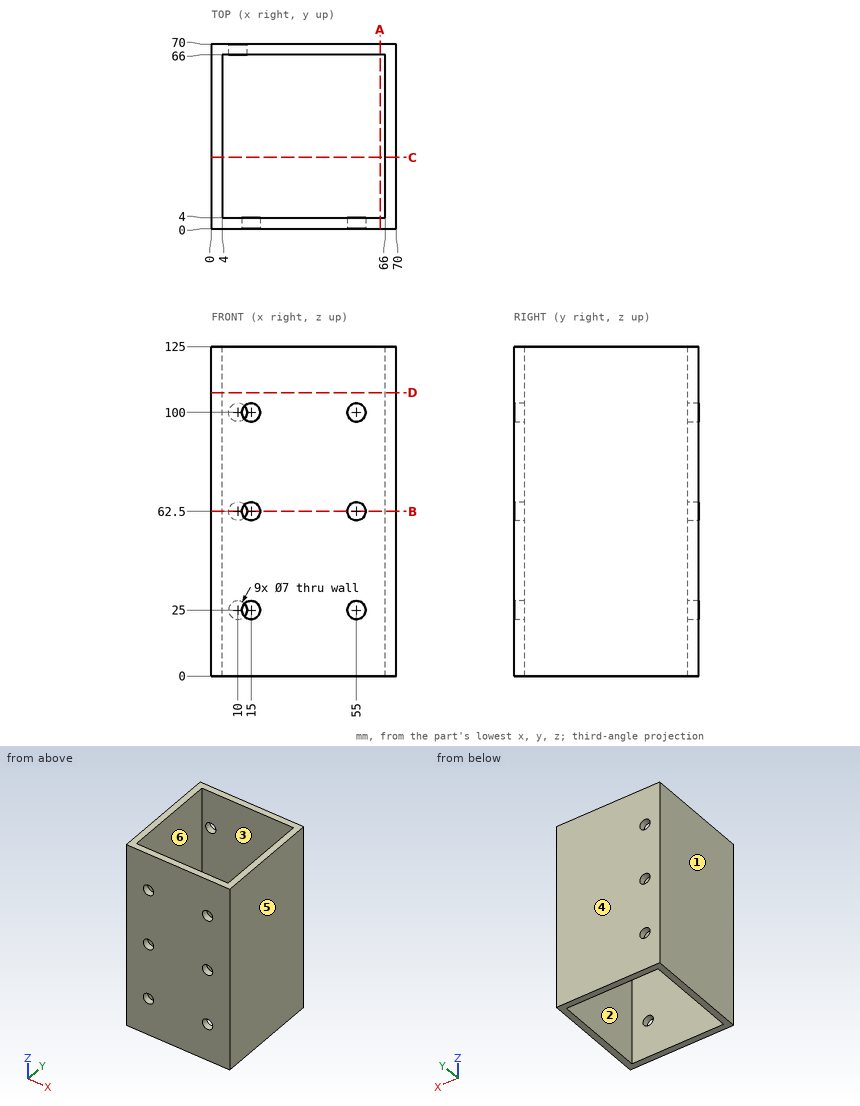
Part print with two shaded views. Sizes in mm from the minimum x, y, z corner. A direction names the side the tool comes from. Coordinates: 2 decimals unless noted, no trailing zeros. Loops run counter-clockwise (first coordinate to the right, second up) from the corner with the lowest first, then second, coordinate; pieces in that order, holes last. Notation, with made-up numbers: (59, 83) -> (101, 83) arc R27 ccw to (101, 104) -> close; hole circle Ø7 at (8, 11). An arc over 180 degrees is marked (long way). Answer as a JSON object with one key per item and string values.
Q1. Flat gauge pins, fed straight in: P1, Ø4, axis at x = 55, z = 62.5, coming from the -Y side; P2, Ø3, axis at x = 42, z = 91.5, coming from the -Y side; P3, Ø10, axis at x = 56.5, y = 50, coming from the +Z side. Where does each tip first touch, or does it go through?
Report:
{"P1": "stops at y = 66", "P2": "stops at y = 0", "P3": "passes through"}
Q2. Probe probe 1 along Z at (x, y) = (15, 2.45); probe 2 along Y at (x, z) = (12, 35); probe 3 along X at (y, z) = (2.8, 100). List the from-to ranges inside material, lowest first.
Report:
{"probe 1": "z = 0 to 21.5, 28.5 to 59, 66 to 96.5, 103.5 to 125", "probe 2": "y = 0 to 4, 66 to 70", "probe 3": "x = 0 to 11.5, 18.5 to 51.5, 58.5 to 70"}
Q3. 3-axis set-ups, long thin cutter, end or side, ignore diameter. For the marked faces 1 and 2: which of +Z, -Z, +X, -X, +Y, -Y reach the whole face in a straight line?
Report:
{"face 1": "+Z, -Z, -X, +Y, -Y", "face 2": "+Z, -Z"}
Q4. Cut at D-D (z = 107.5). List the corners of the cut face in (x, y).
Report:
{"outline": "(0, 0) -> (70, 0) -> (70, 70) -> (0, 70) -> close; hole (4, 4) -> (66, 4) -> (66, 66) -> (4, 66) -> close"}
Q5. Pull direction X, two halves, no side cores. Call the marked faces 3, 4, 5 and 6: released by +X, released by -X, zero draft, split by the parting line, or undercut.
Report:
{"face 3": "undercut", "face 4": "zero draft", "face 5": "released by +X", "face 6": "undercut"}
Q6. Cut at A-A (x = 64). List the corners of the cut face in (y, z).
Report:
{"outline": "(0, 0) -> (4, 0) -> (4, 125) -> (0, 125) -> close; (66, 0) -> (70, 0) -> (70, 125) -> (66, 125) -> close"}
Q7. Cut at B-B (z = 62.5). List the corners of the cut face in (x, y).
Report:
{"outline": "(0, 0) -> (11.5, 0) -> (11.5, 4) -> (4, 4) -> (4, 66) -> (6.5, 66) -> (6.5, 70) -> (0, 70) -> close; (13.5, 66) -> (66, 66) -> (66, 4) -> (58.5, 4) -> (58.5, 0) -> (70, 0) -> (70, 70) -> (13.5, 70) -> close; (18.5, 0) -> (51.5, 0) -> (51.5, 4) -> (18.5, 4) -> close"}
